Could you check a few things on this drawing? It's one solid part, dimensions in mm from its lowest x, y, z. Give positions to 0.01 mm unless a question says otherwise; leave off trailing zeros. Order: outer loops, then holes, each group sorted by start corner. A loop starts at its lowest first (then second) coordinate and runs counter-clockwise, first axis right, second up.
(1) Imagine slicing it at D-D, the plane z = 34.45. Write out the boundary of the cut face in (x, y), then the cut area to 3 significant figures.
(2) If I drill on probe 1 along Z at (x, y) = (31.2, 2.45); probe 2 along X at (y, z) = (0.5, 4.45); probe 3 along Z at (x, y) = (2, 0.4), over which ranges is the centre line in solid material (lowest first)?
(3) Imagine slicing it at C-C, the plane y = 2.5. Write out the boundary of the cut face in (x, z), then the cut area to 3 significant figures.
(4) Will this pin go through, and if not, where does the flat tip stop? pin 1 (1.5 mm diameter, centred on x = 30.5, z = 33.5, fed in from +Y).
(5) Imagine slicing it at A-A, the plane z = 4.45. Write out the boundary of the cut face in (x, y), then the cut area to 3 significant figures.
(6) Imagine slicing it at B-B, the plane x = 2. Write out the boundary of the cut face in (y, z), then the cut area to 4 significant figures.
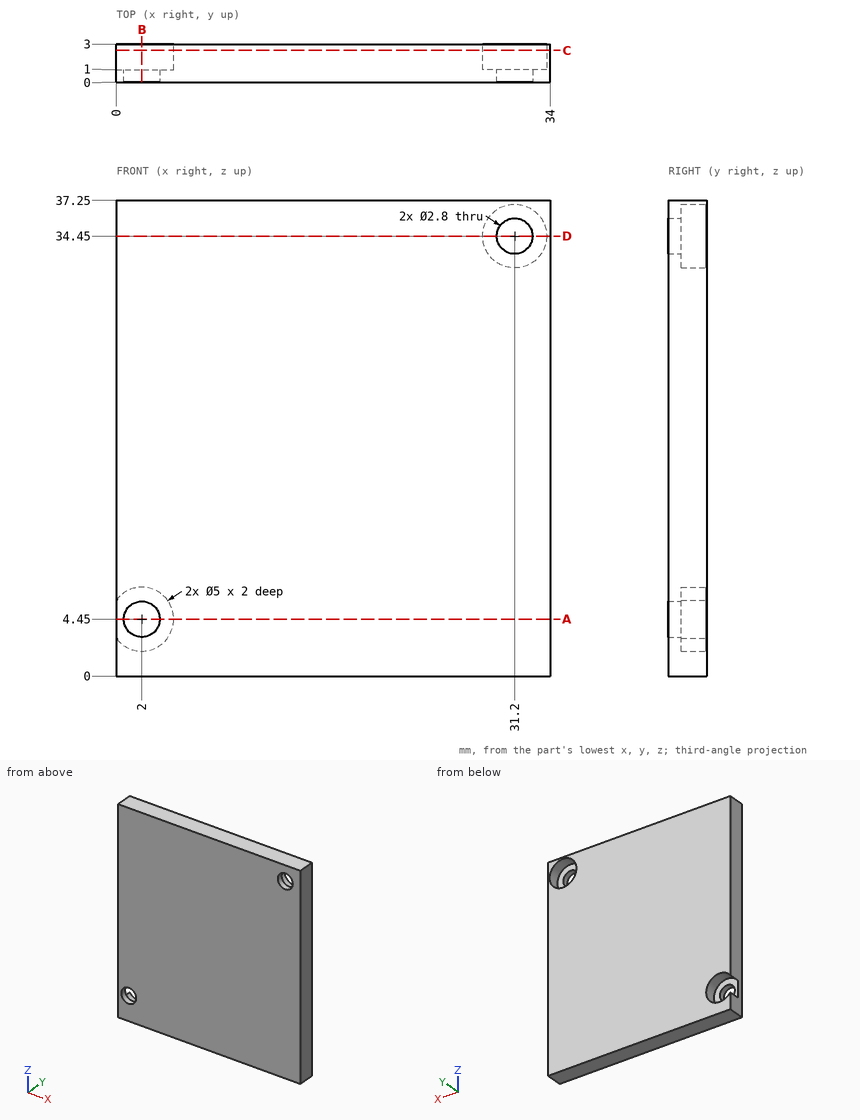
Answer block:
1. outline: (0, 0) - (29.8, 0) - (29.8, 1) - (28.7, 1) - (28.7, 3) - (0, 3) - close; (32.6, 0) - (34, 0) - (34, 3) - (33.7, 3) - (33.7, 1) - (32.6, 1) - close
1. area: 89.2 mm2
2. probe 1: z = 0 to 31.95, 36.95 to 37.25
2. probe 2: x = 0 to 0.6, 3.4 to 34
2. probe 3: z = 0 to 3.05, 5.85 to 37.25
3. outline: (0, 0) - (34, 0) - (34, 37.25) - (0, 37.25) - (0, 5.95) arc R2.5 cw (long way) to (0, 2.95) - close; hole circle Ø5 at (31.2, 34.45)
3. area: 1,230 mm2
4. pin 1: stops at y = 1
5. outline: (0, 0) - (0.6, 0) - (0.6, 1) - (0, 1) - close; (3.4, 0) - (34, 0) - (34, 3) - (4.5, 3) - (4.5, 1) - (3.4, 1) - close
5. area: 90.2 mm2
6. outline: (0, 0) - (3, 0) - (3, 1.95) - (1, 1.95) - (1, 3.05) - (0, 3.05) - close; (0, 5.85) - (1, 5.85) - (1, 6.95) - (3, 6.95) - (3, 37.25) - (0, 37.25) - close
6. area: 98.95 mm2
